Job drawing, mm, ordinate dimensions from the low corner. One solid piece. A direction names the side the tool comes from. Give positions to 0.01 mm unless a question says otherwise; leave off trailing zeros. Order: outer loops, then holes, each group sorted by start corner. A loop starts at its lowest first (then second) coordinate and runs counter-clockwise, first axis right, second up.
1. Probe line 1 (Y direction, x = 6, z = 1); line 2 (Y direction, x = 3.5, z = 5); line 3 (X direction, y = 12, z = 7.25). List the from-to ranges inside material, lowest first.
2. Which spindle directions (+Z, -Z, +X, -X, +Y, -Y) get a long thin tool onto all of the face, cutting with end or side? Do the marked faces 1, 2 and 3. Say none if no direction does.
3. Mould opens along Z. For the marked faces 4, 5 and 6 say: +Z half, -Z half, draft (parallel to the pull), parting line (faces both ways), or undercut.
4. Slice it at D-D on y = 27. List the corners of the cut face in (x, z) (1 decimal), and give its area (3 significant figures).
5. Drop flat-ended pins along their axis: pin 1 Ø2 at (y, z) = (23.5, 4) entering from -X; pin 2 Ø1 at (x, y) = (6, 13.5) entering from +Z; pin 3 Ø3 at (y, z) = (17, 1.5) entering from -X. Give the stop position or say it passes through.
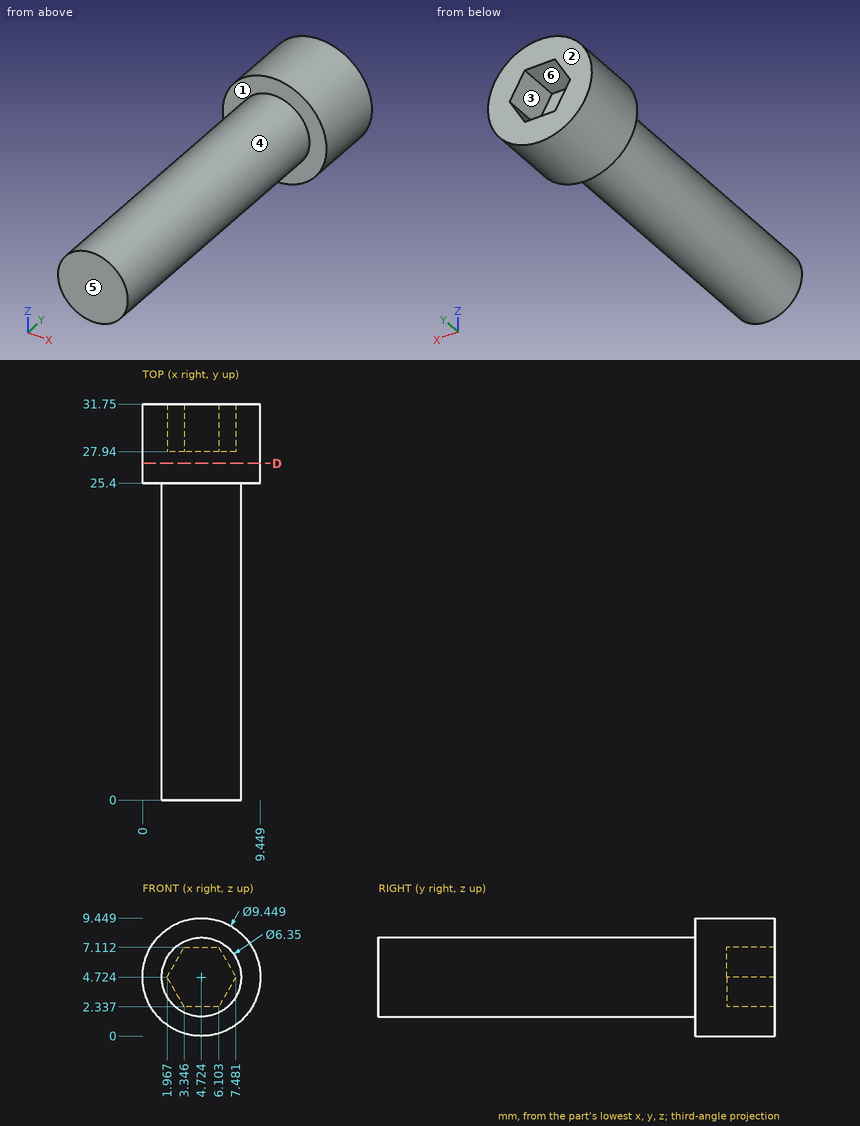
Data:
1. line 1: y = 25.4 to 31.75
1. line 2: y = 0 to 27.94
1. line 3: x = 2.8 to 6.65
2. face 1: -Y
2. face 2: +Z, -Z, +X, -X, +Y
2. face 3: +Y
3. face 4: parting line
3. face 5: draft
3. face 6: undercut
4. outline: circle Ø9.4 at (4.7, 4.7)
4. area: 70.1 mm2
5. pin 1: stops at x = 1.55
5. pin 2: stops at z = 7.8
5. pin 3: stops at x = 2.06
